Design review of the part built by this model. Coordinates are the model's own, in mm. A direction names the side the tool comes from. Coordinates: 2 decimals unless noted, no trailing zeros. Loops run counter-clockwise (first coordinate to the right, second up) from the corner with the lowest first, then second, coordinate; pieces in that order, holes last. Notation, with made-up numbers: (-15, 88.25) -> (36, 88.25) arc R15 cw to (36, 113.25) -> close; hole circle Ø7 at (-33.5, 47.25). An arc over 180 degrees is marked (long way). Answer in a Markdown table with one row per item.
```python
from build123d import *

# Parameters (mm, degrees)
LOCATING_TONGUE_DEPTH = 1
COVER_FLANGE_DEPTH    = 0.9


with BuildPart() as part:
    # Locating_tongue_profile → Locating_tongue (new body)
    with BuildSketch(Plane.XY):
        with BuildLine():
            Line((1, 0), (9.8, 0))
            ThreePointArc((9.8, 0), (10.507106781, 0.292893219), (10.8, 1))
            Line((10.8, 1), (10.8, 2.5))
            ThreePointArc((10.8, 2.5), (10.507106781, 3.207106781), (9.8, 3.5))
            Line((9.8, 3.5), (1, 3.5))
            ThreePointArc((1, 3.5), (0.292893219, 3.207106781), (0, 2.5))
            Line((0, 2.5), (0, 1))
            ThreePointArc((0, 1), (0.292893219, 0.292893219), (1, 0))
        make_face()
    extrude(amount=-LOCATING_TONGUE_DEPTH)

    # Cover_flange_profile → Cover_flange (add)
    with BuildSketch(Plane.XY):
        with BuildLine():
            Line((0, -0.615549442), (0, 4.115549442))
            ThreePointArc((0, 4.115549442), (0.480165382, 4.327504301), (1, 4.4))
            Line((1, 4.4), (9.8, 4.4))
            ThreePointArc((9.8, 4.4), (11.143502884, 3.843502884), (11.7, 2.5))
            Line((11.7, 2.5), (11.7, 1))
            ThreePointArc((11.7, 1), (11.143502884, -0.343502884), (9.8, -0.9))
            Line((9.8, -0.9), (1, -0.9))
            ThreePointArc((1, -0.9), (0.480165382, -0.827504301), (0, -0.615549442))
        make_face()
    extrude(amount=COVER_FLANGE_DEPTH)


solid = part.part
```
(1) For pin 1 (0.8 mm diameter, centred on x = 5.5, z = -0.5, fed in from -Y); pin 2 (0.5 mm diameter, centred on x = 6.5, z = -0.5, fed in from +Y); pin 3 (1.1 mm diameter, centred on y = 1.5, z = -0.5, fed in from +X), all flat-tipped, find the tip position at first contact; note any pin that passes through.
Evaluation:
| item | result |
|---|---|
| pin 1 | stops at y = 0 |
| pin 2 | stops at y = 3.5 |
| pin 3 | stops at x = 11.7 |
(2) Take a section at A-A on x = 7.75. Give the boundary of the cut face in (y, z), and give its area (3 significant figures).
Evaluation:
| item | result |
|---|---|
| outline | (-0.9, 0) -> (0, 0) -> (0, -1) -> (3.5, -1) -> (3.5, 0) -> (4.4, 0) -> (4.4, 0.9) -> (-0.9, 0.9) -> close |
| area | 8.27 mm² |
(3) Take a section at C-C on y = 1.5. Give the boundary of the cut face in (x, z).
Evaluation:
| item | result |
|---|---|
| outline | (0, -1) -> (10.8, -1) -> (10.8, 0) -> (11.7, 0) -> (11.7, 0.9) -> (0, 0.9) -> close |
(4) To check wall thickness, follow probe 1 along X at (y, z) = (2.2, -0.15); probe 2 along Z at (x, y) = (9.5, -0.4); probe 3 along Y at (x, z) = (1.75, -0.05). State the ranges of each line that lie inside material, in increasing order.
Evaluation:
| item | result |
|---|---|
| probe 1 | x = 0 to 10.8 |
| probe 2 | z = 0 to 0.9 |
| probe 3 | y = 0 to 3.5 |
(5) Take a section at B-B on y = 0.5. Give the boundary of the cut face in (x, z).
Evaluation:
| item | result |
|---|---|
| outline | (0, 0) -> (0.13, 0) -> (0.13, -1) -> (10.67, -1) -> (10.67, 0) -> (11.63, 0) -> (11.63, 0.9) -> (0, 0.9) -> close |
(6) Tool access review of faces 1 (the flat face through (5.5, 3.5, -0.5)), 2 (the cylindrical face through (10.515, 3.199, -0.493)), 3 (the cylindrical face through (0.285, 0.301, -0.493)), 4 (the cylindrical face through (0.301, 3.215, -0.493)), 5 (the cylindrical face through (10.499, 0.285, -0.493)): name each direction out of +Z, -Z, +X, -X, +Y, -Y from which nothing blocks a thin tool from reaching the whole face with its end or side.
Evaluation:
| item | result |
|---|---|
| face 1 | -Z, +X, -X, +Y |
| face 2 | -Z, +X, +Y |
| face 3 | -Z, -X, -Y |
| face 4 | -Z, -X, +Y |
| face 5 | -Z, +X, -Y |
(7) Take a section at D-D on y = -0.3. Give the boundary of the cut face in (x, z), and give its area (3 significant figures).
Evaluation:
| item | result |
|---|---|
| outline | (0, 0) -> (11.19, 0) -> (11.19, 0.9) -> (0, 0.9) -> close |
| area | 10.1 mm² |
